from build123d import *

# Parameters (mm, degrees)
BOSS_EXTRUDE1_DEPTH = 40
SKETCH16_R          = 3.5
CUT_EXTRUDE5_DEPTH  = 96.547228328
SKETCH17_R          = 4
CUT_EXTRUDE7_DEPTH  = 96.547228328
FILLET1_R           = 5


with BuildPart() as part:
    # Sketch1 → Boss-Extrude1 (new, symmetric)
    with BuildSketch(Plane.XY):
        Polygon((0, -23.280493307), (0, 86.719506693), (3, 86.719506693), (3, 83.719506693), (3, -23.280493307), align=None)
    extrude(amount=BOSS_EXTRUDE1_DEPTH, both=True)

    # Sketch16 → Cut-Extrude5 (cut, through all)
    with BuildSketch(Plane(origin=(3, 0, 0), x_dir=(0, 0, -1), z_dir=(1, 0, 0))):
        with Locations((-19.5, 11.719506693)):
            Circle(SKETCH16_R)
        with Locations((19.5, 11.719506693)):
            Circle(SKETCH16_R)
        with Locations((19.5, 41.719506693)):
            Circle(SKETCH16_R)
        with Locations((-19.5, 41.719506693)):
            Circle(SKETCH16_R)
    extrude(amount=-CUT_EXTRUDE5_DEPTH, mode=Mode.SUBTRACT)

    # Sketch17 → Cut-Extrude7 (cut, through all)
    with BuildSketch(Plane.ZY):
        with Locations((-25, 66.719506693)):
            Circle(SKETCH17_R)
        with Locations((24.997500187, 66.719506693)):
            Circle(SKETCH17_R)
        with Locations((-25, -13.280493307)):
            Circle(SKETCH17_R)
        with Locations((24.997500187, -13.280493307)):
            Circle(SKETCH17_R)
    extrude(amount=-CUT_EXTRUDE7_DEPTH, mode=Mode.SUBTRACT)

    # Fillet1
    fillet1_edges = [part.edges().sort_by_distance(p)[0] for p in [
        (1.5, 86.719506693, 40),
        (1.5, -23.280493307, 40),
        (1.5, 86.719506693, -40),
        (1.5, -23.280493307, -40),
    ]]
    fillet(fillet1_edges, radius=FILLET1_R)


solid = part.part
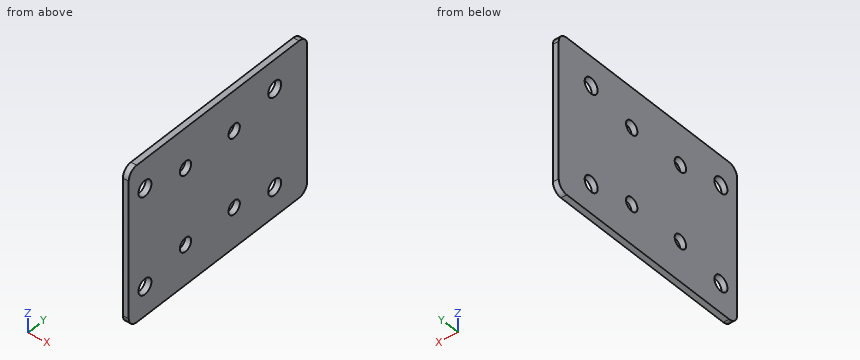
Check sheet for the modelled part. Datum: model origin and axes. Units: mm. Give positions to 0.01 mm unless a question says otherwise; leave off trailing zeros. Loops run counter-clockwise (first coordinate to the right, second up) from the corner with the lowest first, then second, coordinate; pieces in that order, holes last. Notation, with made-up numbers: M 3,-1 L 16,-1 A19 cw 16,31 Z; hole C 60,77.25 d6. An arc over 180 degrees is marked long. Use a Markdown table: item, result. Add a question column.
Q1. Sectioned sample at B-B, the plane y = 9.5. Record the cut outline in (x, z), then the cut area to 3 significant figures.
Q2. Sectioned sample at C-C, the plane x = 1.75. Give the number of separate pieces and of enclosed holes in the cut face, then the cut area to 3 significant figures.
Q3. Go/stop test with flat-tipped pins: pin 1 (7 mm diameter, centred on y = -13.28, z = -25, fed in from -X); pin 2 (3 mm diameter, centred on y = 63.5, z = -12, fed in from -X). Record where each tip stops, or that it passes through.
Q4. Sectioned sample at A-A, the plane z = -25. Record the cut outline in (x, y), then the cut area to 3 significant figures.
Q5. Scan lines: line 1 along Y through (x, z) = (1.7, 19.5); line 2 along Y through (x, z) = (0.35, -24.5); line 3 along Z through (x, y) = (1, 41). Record each from-to range of solid material in increasing order. Write a range as [from, to].
Verdict:
| question | item | result |
|---|---|---|
| 1 | outline | M 0,-40 L 3,-40 L 3,-22.21 L 0,-22.21 Z; M 0,-16.79 L 3,-16.79 L 3,16.79 L 0,16.79 Z; M 0,22.21 L 3,22.21 L 3,40 L 0,40 Z |
| 1 | area | 208 mm^2 |
| 2 | separate pieces | 1 |
| 2 | enclosed holes | 8 |
| 2 | area | 8,420 mm^2 |
| 3 | pin 1 | through |
| 3 | pin 2 | x = 0 |
| 4 | outline | M 0,-23.28 L 3,-23.28 L 3,-17.28 L 0,-17.28 Z; M 0,-9.28 L 3,-9.28 L 3,62.72 L 0,62.72 Z; M 0,70.72 L 3,70.72 L 3,86.72 L 0,86.72 Z |
| 4 | area | 282 mm^2 |
| 5 | line 1 | [-23.28, 8.22], [15.22, 38.22], [45.22, 86.72] |
| 5 | line 2 | [-23.28, -17.25], [-9.31, 62.75], [70.69, 86.72] |
| 5 | line 3 | [-40, -22.93], [-16.07, 16.07], [22.93, 40] |
